Geometry: see drawing. Coordinates: mm, zero at the bounding-box minimum. A direction names the side the tool comes from. Coordinates: 2 decimals unless noted, no trailing zeros. Write each loop counter-clockwise with the first axis right and the second up, starting at its lowest first coordinate (ties: lowest second). Pieces come first, ordered by that corner, then holes. Notation, with made-up numbers: M -32,32 L 14,32 A22 cw 14,54 Z; hole C 51.25,22 d2. An arc over 180 degrees is marked long. One line per item, written item: value. Start each with the question number.
Item 1: Cut plane B-B, the plane y = 24. Output: boundary loops of the cut face in (x, z).
Item 2: Cut plane D-D, the plane z = 30. Output: boundary loops of the cut face in (x, y) (3 decimals).
Item 3: Cut plane A-A, the plane y = 12.95. Output: boundary loops of the cut face in (x, z).
Item 4: Pin query (flat end, axial travel): P1, Ø11.5, axis at x = 34.5, z = 12, coming from the -Y side; P2, Ø1, axis at y = 16.5, z = 17.5, coming from the -X side; P3, Ø5, axis at x = 6, y = 5, coming from the -Z side. Return the tip coordinate at first contact, or that it passes through.
Item 5: Set-up query: the marked faces 1, 2 and 3. Return all of +Z, -Z, +X, -X, +Y, -Y with unobstructed straight access to the full face (end or side cutting, diameter ignored); none if empty.
Item 6: Ray query, L1, parallel to Y at x = 28, z = 5.5 (3 decimals); L2, parallel to Z at x = 51, y = 8; L3, parallel to Z at x = 20.5, y = 10.5. Return the intervals inside material, ascending. Write a range as from..to.
Item 7: Cut plane C-C, the plane x = 52. Output: boundary loops of the cut face in (y, z) (3 decimals), then the cut area to 3 significant figures.
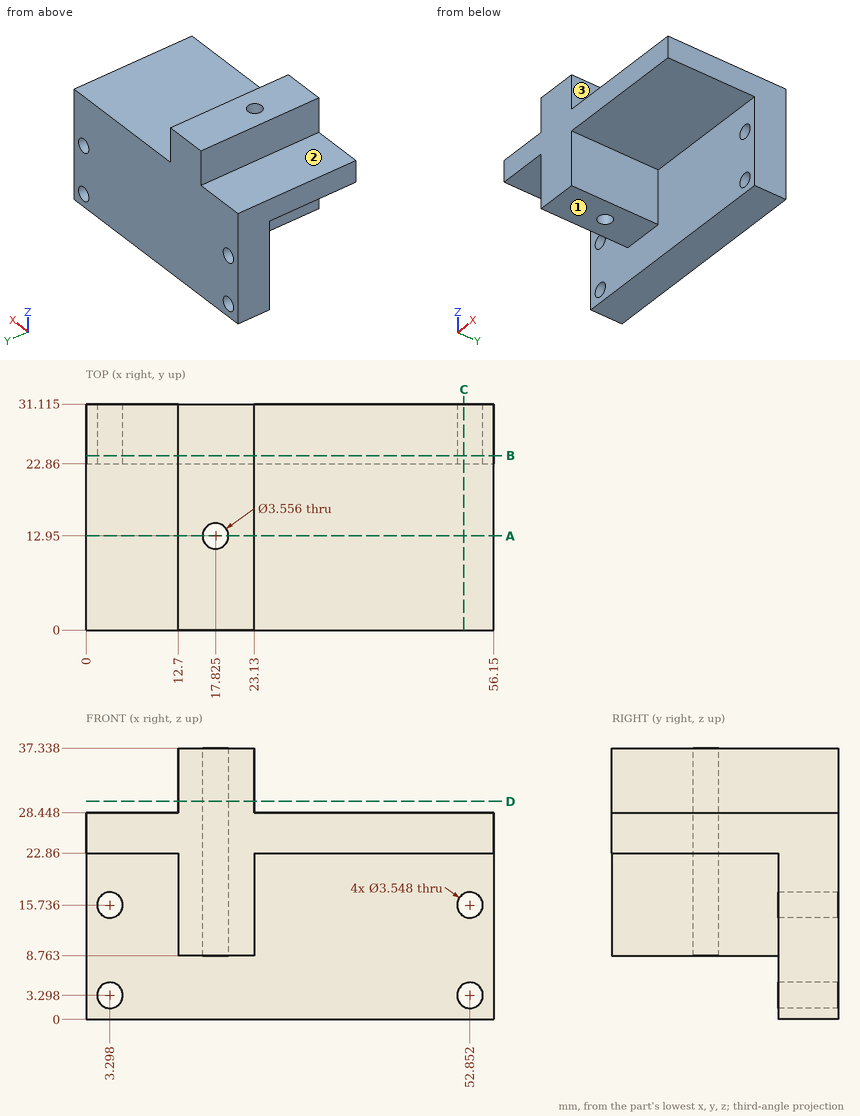
From the geometry:
1. outline: M 0,0 L 56.15,0 L 56.15,28.45 L 23.13,28.45 L 23.13,37.34 L 12.7,37.34 L 12.7,28.45 L 0,28.45 Z; hole C 3.3,3.3 d3.55; hole C 3.3,15.74 d3.55; hole C 52.85,3.3 d3.55; hole C 52.85,15.74 d3.55
2. outline: M 12.7,0 L 23.13,0 L 23.13,31.115 L 12.7,31.115 Z; hole C 17.825,12.95 d3.556
3. outline: M 0,22.86 L 12.7,22.86 L 12.7,8.76 L 16.05,8.76 L 16.05,37.34 L 12.7,37.34 L 12.7,28.45 L 0,28.45 Z; M 19.6,8.76 L 23.13,8.76 L 23.13,22.86 L 56.15,22.86 L 56.15,28.45 L 23.13,28.45 L 23.13,37.34 L 19.6,37.34 Z
4. P1: stops at y = 22.86
4. P2: stops at x = 12.7
4. P3: stops at z = 22.86
5. face 1: -Z, +X, -X, -Y
5. face 2: +Z, -X, +Y, -Y
5. face 3: +Z, +X, +Y, -Y
6. L1: y = 22.86..31.115
6. L2: z = 22.86..28.45
6. L3: z = 8.76..37.34
7. outline: M 0,22.86 L 22.86,22.86 L 22.86,17.292 L 31.115,17.292 L 31.115,28.448 L 0,28.448 Z; M 22.86,0 L 31.115,0 L 31.115,1.742 L 22.86,1.742 Z; M 22.86,4.854 L 31.115,4.854 L 31.115,14.18 L 22.86,14.18 Z
7. area: 311 mm²
